from build123d import *

# Parameters (mm, degrees)
F2_R     = 7.5
F3_DEPTH = 30
F4_DEPTH = 3
F5_R     = 7.5
F6_DEPTH = 33
F7_R     = 7.5
F8_DEPTH = 33


with BuildPart() as f1:
    # F0 (on Front) → F1 (revolve)
    with BuildSketch(Plane.XZ):
        with BuildLine():
            Line((0, 39), (0, 31))
            Line((0, 31), (30, 29))
            Line((30, 29), (30, 23.2778316429))
            Line((30, 23.2778316429), (72, 23.2778316429))
            Line((72, 23.2778316429), (72, 0))
            Line((72, 0), (90, 0))
            Line((90, 0), (90, 42))
            Line((90, 42), (93, 42))
            Line((93, 42), (93, 52))
            Line((93, 52), (60, 52))
            Line((60, 52), (60, 42.5))
            Line((60, 42.5), (45.9028487651, 32.629068438))
            ThreePointArc((45.9028487651, 32.629068438), (45.8614157942, 32.5997709837), (45.8197142818, 32.5708570462))
            ThreePointArc((45.8197142818, 32.5708570462), (41.5456906901, 31.7290536585), (38, 34.2596638885))
            Line((38, 34.2596638885), (38, 45))
            Line((38, 45), (8, 45))
            Line((8, 45), (8, 39))
            Line((8, 39), (0, 39))
        make_face()
    revolve(axis=Axis((81, 0, 0), (-1, 0, 0)))

    # F2 (on face) → F3 (join)
    with BuildSketch(Plane.YZ.offset(90)):
        with BuildLine():
            Line((-19.1190099356, 37.3960353391), (-80.8199036363, 16.2655922909))
            ThreePointArc((-80.8199036363, 16.2655922909), (-90, 0), (-80.8199036363, -16.2655922909))
            Line((-80.8199036363, -16.2655922909), (-19.1190099356, -37.3960353391))
            ThreePointArc((-19.1190099356, -37.3960353391), (-42, 0), (-19.1190099356, 37.3960353391))
        make_face()
        with Locations((-71, 0)):
            Circle(F2_R, mode=Mode.SUBTRACT)
        with BuildLine():
            Line((80.8199036363, 16.2655922909), (19.1190099356, 37.3960353391))
            ThreePointArc((19.1190099356, 37.3960353391), (35.825957191, 21.9203282674), (42, 0))
            ThreePointArc((42, 0), (35.825957191, -21.9203282674), (19.1190099356, -37.3960353391))
            Line((19.1190099356, -37.3960353391), (80.8199036363, -16.2655922909))
            ThreePointArc((80.8199036363, -16.2655922909), (90, 0), (80.8199036363, 16.2655922909))
        make_face()
        with Locations((71, 0)):
            Circle(F2_R, mode=Mode.SUBTRACT)
        with Locations((-71, 0)):
            Circle(F2_R)
        with Locations((71, 0)):
            Circle(F2_R)
    extrude(amount=-F3_DEPTH)

    # F4 (add): faces of the model
    f4_faces = [f1.faces().sort_by_distance(p)[0] for p in [
        (90, 66.461472241, 0),
        (90, -66.461472241, 0),
    ]]
    extrude(f4_faces, amount=F4_DEPTH)

    # F5 (on face) → F6 (cut)
    with BuildSketch(Plane(origin=(60, 0, 0), x_dir=(0, -1, 0), z_dir=(-1, 0, 0))):
        with Locations((-71, 0)):
            Circle(F5_R)
    extrude(amount=-F6_DEPTH, mode=Mode.SUBTRACT)

    # F7 (on face) → F8 (cut)
    with BuildSketch(Plane(origin=(60, 0, 0), x_dir=(0, -1, 0), z_dir=(-1, 0, 0))):
        with Locations((71, 0)):
            Circle(F7_R)
    extrude(amount=-F8_DEPTH, mode=Mode.SUBTRACT)


solid = f1.part
Work out the finished part from the listing and answer in its coordinate system (mm). A direction names the side the tool comes from. Round coordinates to 2 decimals unless told otherwise and drop trailing zeros. Write each loop counter-clockwise with the first axis right and the second up, starting at its lowest first coordinate (ties: lowest second). Pieces come first, ordered by that corner, then holes. Notation, with made-up numbers: (32, -3.75) -> (64, -3.75) arc R18 ccw to (64, 1.25) -> close; hole circle Ø11 at (-37.5, -18.75). An arc over 180 degrees is marked (long way). Write each question's results on one line, items separated by ' | '.
Item 1: Flat-ended cylindrical pins translate along their axes: P1, Ø10, axis at x = 16.5, z = 4.5, coming from the -Y side; P2, Ø1, axis at y = 19, z = -2, coming from the -X side; P3, Ø12, axis at x = 45.5, y = -5.5, coming from the -Z side; P4, Ø1.5, axis at x = 42.5, z = 32.5, coming from the -Y side (3 decimals). Find the tip coordinate at first contact, or state that the pin passes through.
Result set:
P1: y = -45 | P2: x = 72 | P3: z = -36.21 | P4: through
Item 2: Which of the six approach directions +Z, -Z, +X, -X, +Y, -Y give full straight-line access (tool end or side, diameter ignored) to faces 4 (the face through (0, -17.2, -26.2)), 5 (the face through (91.52, 12.62, 40.06)), 6 (the face through (8, 37, -14)), 7 (the face through (60, 0, -43)), 8 (the face through (93, 20, -38))?
Result set:
face 4: +Z, -Z, -X, +Y, -Y | face 5: +X | face 6: -X | face 7: none | face 8: +Z, -Z, +X, +Y, -Y
Item 3: The mould has two halves that part along X. Classify faces 1 (the face through (76.73, -62.18, -22.65)), 2 (the face through (72, 0, 0)), 3 (the face through (38, -33, 10)): +X half, -X half, draft (parallel to the pull), parting line (faces both ways), or undercut.
Result set:
face 1: draft | face 2: -X half | face 3: undercut
Item 4: A cutting plane is placed at D-D, the plane y = 71. Determine the outline of the cut face in (x, z), plus the area to 3 significant figures.
Result set:
outline: (60, -19.63) -> (93, -19.63) -> (93, -7.5) -> (60, -7.5) -> close; (60, 7.5) -> (93, 7.5) -> (93, 19.63) -> (60, 19.63) -> close | area: 800 mm^2
Item 5: A cutting plane is placed at A-A, the plane x = 87.5. Determine the outline of the cut face in (y, z).
Result set:
outline: (-80.82, -16.27) -> (-43.02, -29.21) arc R52 ccw to (43.02, -29.21) -> (80.82, -16.27) arc R19 ccw to (80.82, 16.27) -> (43.02, 29.21) arc R52 ccw to (-43.02, 29.21) -> (-80.82, 16.27) arc R19 ccw to start; hole circle Ø15 at (-71, 0); hole circle Ø15 at (71, 0)
Item 6: Find the intervals of material crossed by line 1 along Z through (x, y) = (91.3, 0); line 2 along X through (y, z) = (75, -9); line 3 along Z through (x, y) = (13.5, 27), in increasing order. Write a range as [from, to].
Result set:
line 1: [-52, -42], [42, 52] | line 2: [60, 93] | line 3: [-36, -13.3], [13.3, 36]
Item 7: A cutting plane is placed at B-B, the plane x = 66. Determine the outline of the cut face in (y, z), plus the area to 3 significant figures.
Result set:
outline: (-80.82, -16.27) -> (-43.02, -29.21) arc R52 ccw to (43.02, -29.21) -> (80.82, -16.27) arc R19 ccw to (80.82, 16.27) -> (43.02, 29.21) arc R52 ccw to (-43.02, 29.21) -> (-80.82, 16.27) arc R19 ccw to start; hole circle Ø15 at (-71, 0); hole circle Ø46.56 at (0, 0); hole circle Ø15 at (71, 0) | area: 9,590 mm^2
Item 8: A cutting plane is placed at C-C, the plane y = -70. Determine the outline of the cut face in (x, z).
Result set:
outline: (60, -19.97) -> (93, -19.97) -> (93, -7.43) -> (60, -7.43) -> close; (60, 7.43) -> (93, 7.43) -> (93, 19.97) -> (60, 19.97) -> close
